Can you work these out from the drawing? Everything is in mm from the part's minimum corner. A direction names the side the tool comes from. Coordinates: 2 decimals unless noted, no trailing zeros. Order: outer loops, then holes, each group sorted by start corner. A loop starts at its lowest first (then second) coordinate and runs counter-clockwise, first axis right, second up. Notation, with made-up numbers: (76, 39.5) - (95, 39.5) arc R5 ccw to (95, 45.5) - close; hole circle Ø3 at (65, -27.5). An arc over 180 degrees is marked (long way). One line per item, written item: value.
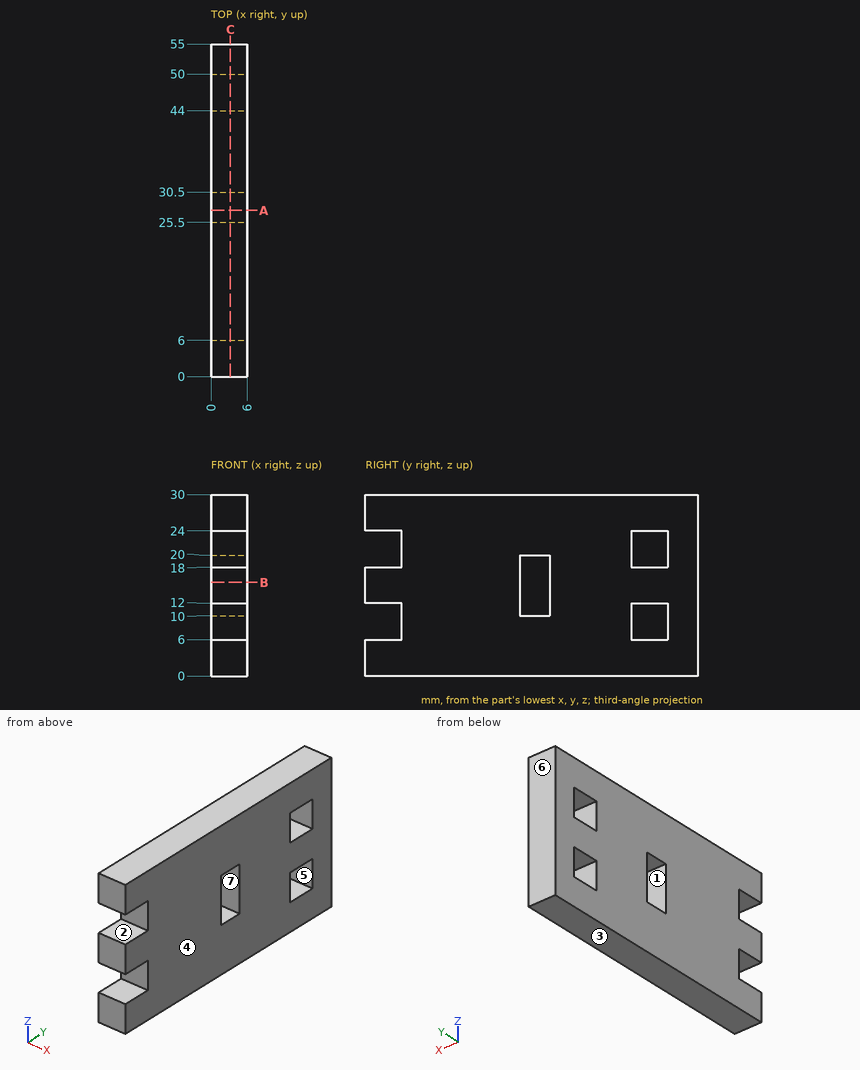
Item 1: I want a section at C-C on x = 3.2. Please give me the cut outline in (y, z).
Conclusion:
outline: (0, 0) - (55, 0) - (55, 30) - (0, 30) - (0, 24) - (6, 24) - (6, 18) - (0, 18) - (0, 12) - (6, 12) - (6, 6) - (0, 6) - close; hole (25.5, 10) - (30.5, 10) - (30.5, 20) - (25.5, 20) - close; hole (44, 6) - (50, 6) - (50, 12) - (44, 12) - close; hole (44, 18) - (50, 18) - (50, 24) - (44, 24) - close
Item 2: If I drill on probe 1 along Z at (x, y) = (1.45, 3); probe 2 along Y at (x, z) = (1.05, 11.75); probe 3 along Y at (x, z) = (3.9, 8.5), over which ranges is the centre line in solid material (lowest first)?
Conclusion:
probe 1: 0 to 6, 12 to 18, 24 to 30
probe 2: 6 to 25.5, 30.5 to 44, 50 to 55
probe 3: 6 to 44, 50 to 55
Item 3: I want a section at B-B on z = 15.5. Please give me the cut outline in (x, y), then the cut area to 3 significant figures.
Conclusion:
outline: (0, 0) - (6, 0) - (6, 25.5) - (0, 25.5) - close; (0, 30.5) - (6, 30.5) - (6, 55) - (0, 55) - close
area: 300 mm²
Item 4: Thinking about a two-plate mould opening in Y: for the marked faces 4, 5, 6 and 7, which applies, pulls with the +Y half, pulls with the -Y half, needs draft (parallel to the pull), parting line crosses it, or undercut?
Conclusion:
face 4: needs draft
face 5: undercut
face 6: pulls with the +Y half
face 7: undercut
Item 5: I'm going to push a flat-ended pin straight in: pin 1 Ø3 at (x, z) = (1.5, 8) entering from -Y. Where does the tip first touch, or does it pass through?
Conclusion:
pin 1: y = 6
Item 6: I want a section at A-A on y = 27.5. Please give me the cut outline in (x, z).
Conclusion:
outline: (0, 0) - (6, 0) - (6, 10) - (0, 10) - close; (0, 20) - (6, 20) - (6, 30) - (0, 30) - close
Item 7: For the marked faces 1, 2 and 3, which set-ups out of +Z, -Z, +X, -X, +Y, -Y let a thin tool reach every point of the face, with its end or its side?
Conclusion:
face 1: +X, -X
face 2: +X, -X, -Y
face 3: -Z, +X, -X, +Y, -Y
